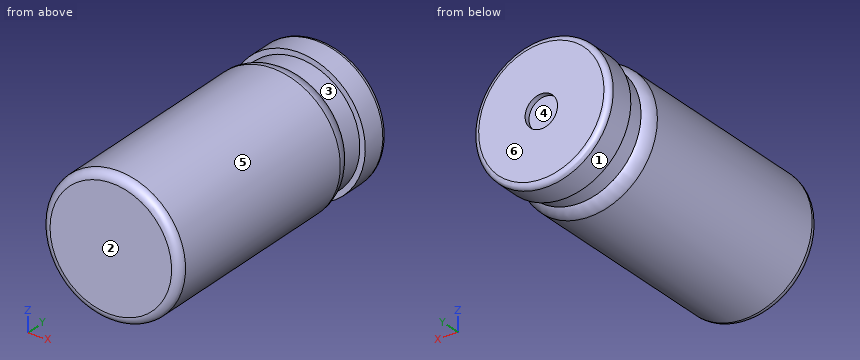
```python
from build123d import *

# Parameters (mm, degrees)
FILLET1_R = 3.5
FILLET2_R = 1.5
FILLET3_R = 1


with BuildPart() as part:
    # Sketch1 → Revolve1 (revolve)
    with BuildSketch(Plane.XY):
        Polygon((0, 0), (-12.745, 0), (-12.745, 43.73), (-11.595, 43.73), (-11.595, 51.23), (0, 51.23), align=None)
    revolve(axis=Axis((0, 51.23, 0), (0, -1, 0)))

    # Fillet1
    # the kernel refuses this fillet: 3.5 mm, written as the material it takes off along each edge
    with BuildSketch(Plane(origin=(0, 43.73, 0), x_dir=(-1, 0, 0), z_dir=(0, 0, 1))) as fillet1_piece_1:
        with BuildLine():
            CenterArc((9.245, 2.59374247), FILLET1_R, 312.177418601, 47.822581399)
            Line((11.595, 0), (11.642, -0.051874849))
            ThreePointArc((11.642, -0.051874849), (12.17, -0.07), (12.745, -0.07))
            Line((12.745, -0.07), (12.815, 0))
            Line((12.815, 0), (12.815, 2.59374247))
            Line((12.815, 2.59374247), (12.745, 2.59374247))
        make_face()
    revolve(axis=Axis((0, 43.73, 0), (0, -1, 0)), mode=Mode.SUBTRACT)

    # Fillet2
    fillet2_edges = [part.edges().sort_by_distance(p)[0] for p in [
        (12.745, 0, 0),
    ]]
    fillet(fillet2_edges, radius=FILLET2_R)

    # Sketch2 → Revolve2 (revolve)
    with BuildSketch(Plane(origin=(0, 0, 0), x_dir=(0, 0, -1), z_dir=(1, 0, 0)), mode=Mode.PRIVATE) as revolve2_sk:
        Polygon((3, 52.23), (11.595, 52.23), (11.595, 47.73), (12.595, 47.73), (12.595, 53.23), (3, 53.23), align=None)
    revolve(revolve2_sk.sketch.rotate(Axis((0, 51.23, 0), (0, -1, 0)), 180), axis=Axis((0, 51.23, 0), (0, -1, 0)))

    # Fillet3
    fillet3_edges = [part.edges().sort_by_distance(p)[0] for p in [
        (0, 53.23, -12.595),
    ]]
    fillet(fillet3_edges, radius=FILLET3_R)


solid = part.part
```
Check sheet for the modelled part. Datum: model origin and axes. Units: mm. Face numbers are marked on the shaded views. A direction names the side the tool comes from. Give positions to 0.01 mm unless a question says otherwise; leave off trailing zeros. Order: outer loops, then holes, each group sorted by start corner. A loop starts at its lowest first (then second) coordinate and runs counter-clockwise, first axis right, second up. Notation, with made-up numbers: (32.25, -5.75) -> (51.25, -5.75) arc R33 ccw to (51.25, 22.25) -> close; hole circle Ø10 at (-37, -3.75). An arc over 180 degrees is marked (long way). Use CSV: the item, a comma, the result in double quotes. Start each with the question number.
1) Mould release check, pull along Y, two halves, no side actions. Record for the marked faces 4, 5 and 6: released by +Y, released by -Y, zero draft, split by the parting line, or undercut.
2) Go/stop test with flat-tipped pins: P1, Ø1, axis at x = -10, y = 24, coming from the -Z side; P2, Ø1.5, axis at y = 7.5, z = 8, coming from the +X side; P3, Ø4, axis at y = 11, z = -5, coming from the -X side. Record where each tip stops, or that it passes through.
3) Sectioned sample at D-D, the plane y = 49.5. Record the boundary of the cut face in (x, z) (3 decimals), plus the area to 3 significant figures.
4) Sectioned sample at B-B, the plane x = 0. Record the boundary of the cut face in (y, z) (3 decimals).
5) Material ranges on line 1 (Y direction, x = 7, z = 4); line 2 (X direction, y = 52, z = 0) (3 decimals); line 3 (Z direction, x = -0.25, y = 34), recorded low to high. Write a range as from..to.
6) Sectioned sample at A-A, the plane z = 0. Record the boundary of the cut face in (x, y) (3 decimals).
7) Set-up check for the marked faces 1, 2 and 3: record each of +Z, -Z, +X, -X, +Y, -Y from which the full face is reachable in a straight line by a thin tool's end or side.
8) Sectioned sample at C-C, the plane y = 37.5. Record the boundary of the cut face in (x, z) (3 decimals).
Recorded:
1,face 4,"undercut"
1,face 5,"zero draft"
1,face 6,"released by +Y"
2,P1,"z = -8.5"
2,P2,"x = 10.48"
2,P3,"x = -12.39"
3,outline,"circle Ø25.19 at (0, 0)"
3,area,"498 mm2"
4,outline,"(0, -11.245) arc R1.5 ccw to (1.5, -12.745) -> (41.136, -12.745) arc R3.5 ccw to (43.73, -11.595) -> (47.73, -11.595) -> (47.73, -12.595) -> (52.23, -12.595) arc R1 ccw to (53.23, -11.595) -> (53.23, -3) -> (52.23, -3) -> (52.23, -11.595) -> (51.23, -11.595) -> (51.23, 11.595) -> (52.23, 11.595) -> (52.23, 3) -> (53.23, 3) -> (53.23, 11.595) arc R1 ccw to (52.23, 12.595) -> (47.73, 12.595) -> (47.73, 11.595) -> (43.73, 11.595) arc R3.5 ccw to (41.136, 12.745) -> (1.5, 12.745) arc R1.5 ccw to (0, 11.245) -> close"
5,line 1,"0..51.23, 52.23..53.23"
5,line 2,"-12.595..-11.595, 11.595..12.595"
5,line 3,"-12.74..12.74"
6,outline,"(-12.745, 1.5) arc R1.5 ccw to (-11.245, 0) -> (11.245, 0) arc R1.5 ccw to (12.745, 1.5) -> (12.745, 41.136) arc R3.5 ccw to (11.595, 43.73) -> (11.595, 47.73) -> (12.595, 47.73) -> (12.595, 52.23) arc R1 ccw to (11.595, 53.23) -> (3, 53.23) -> (3, 52.23) -> (11.595, 52.23) -> (11.595, 51.23) -> (-11.595, 51.23) -> (-11.595, 52.23) -> (-3, 52.23) -> (-3, 53.23) -> (-11.595, 53.23) arc R1 ccw to (-12.595, 52.23) -> (-12.595, 47.73) -> (-11.595, 47.73) -> (-11.595, 43.73) arc R3.5 ccw to (-12.745, 41.136) -> close"
7,face 1,"+Y"
7,face 2,"+Z, -Z, +X, -X, -Y"
7,face 3,"none"
8,outline,"circle Ø25.49 at (0, 0)"
